```python
from build123d import *

# Parameters (mm, degrees)
SKETCH1_W           = 72
SKETCH1_H           = 36
BOSS_EXTRUDE1_DEPTH = 17
SKETCH2_W           = 124
SKETCH2_H           = 24
BOSS_EXTRUDE2_DEPTH = 12
SKETCH3_W           = 30
SKETCH3_H           = 38
BOSS_EXTRUDE3_DEPTH = 15
SKETCH4_W           = 56
SKETCH4_H           = 34
BOSS_EXTRUDE4_DEPTH = 17
SKETCH5_W           = 38
SKETCH5_H           = 18
CUT_EXTRUDE1_DEPTH  = 10
SKETCH6_R           = 7.25
CUT_EXTRUDE2_DEPTH  = 334.282162739
SKETCH7_R           = 7.5
CUT_EXTRUDE3_DEPTH  = 334.282162739


with BuildPart() as part:
    # Sketch1 → Boss-Extrude1 (new, symmetric)
    with BuildSketch(Plane.XY):
        with Locations((16, 200)):
            Rectangle(SKETCH1_W, SKETCH1_H)
    extrude(amount=BOSS_EXTRUDE1_DEPTH, both=True)

    # Sketch2 → Boss-Extrude2 (add, symmetric)
    with BuildSketch(Plane.XY):
        with Locations((110, 202)):
            Rectangle(SKETCH2_W, SKETCH2_H)
    extrude(amount=BOSS_EXTRUDE2_DEPTH, both=True)

    # Sketch3 → Boss-Extrude3 (add, symmetric)
    with BuildSketch(Plane.XY):
        with Locations((183, 203)):
            Rectangle(SKETCH3_W, SKETCH3_H)
    extrude(amount=BOSS_EXTRUDE3_DEPTH, both=True)

    # Sketch4 → Boss-Extrude4 (add, symmetric)
    with BuildSketch(Plane.XY):
        with Locations((220, 203)):
            Rectangle(SKETCH4_W, SKETCH4_H)
    extrude(amount=BOSS_EXTRUDE4_DEPTH, both=True)

    # Sketch5 → Cut-Extrude1 (cut, symmetric)
    with BuildSketch(Plane.XY):
        with Locations((233, 203)):
            Rectangle(SKETCH5_W, SKETCH5_H)
    extrude(amount=CUT_EXTRUDE1_DEPTH, both=True, mode=Mode.SUBTRACT)

    # Sketch6 → Cut-Extrude2 (cut, through all)
    with BuildSketch(Plane.XY):
        with Locations((0, 198)):
            Circle(SKETCH6_R)
    extrude(amount=-CUT_EXTRUDE2_DEPTH, mode=Mode.SUBTRACT)

    # Sketch7 → Cut-Extrude3 (cut, through all)
    with BuildSketch(Plane.XY):
        with Locations((110, 202)):
            Circle(SKETCH7_R)
    extrude(amount=-CUT_EXTRUDE3_DEPTH, mode=Mode.SUBTRACT)


solid = part.part
```
Verification items for the finished model (mm, model axes). A direction names the side the tool comes from. Give positions to 0.01 mm unless a question says otherwise; leave off trailing zeros. Loops run counter-clockwise (first coordinate to the right, second up) from the corner with the lowest first, then second, coordinate; pieces in that order, holes last. Notation, with made-up numbers: M -2,4 L 17,4 A24 ccw 17,40 Z; hole C 50,36 d7. An arc over 180 degrees is marked long. One line per question, with ' | ' between items.
Item 1: Section check C-C, the plane y = 202. Record the cut outline in (x, z).
Completed:
outline: M -20,-17 L -6.05,-17 L -6.05,0 L 6.05,0 L 6.05,-17 L 52,-17 L 52,-12 L 102.5,-12 L 102.5,0 L 117.5,0 L 117.5,-12 L 168,-12 L 168,-15 L 192,-15 L 192,-17 L 248,-17 L 248,-10 L 214,-10 L 214,10 L 248,10 L 248,17 L 192,17 L 192,15 L 168,15 L 168,12 L 52,12 L 52,17 L -20,17 Z
Item 2: Depth check by flat-ended pin: P1, Ø6, axis at x = 143.5, z = -4.5, coming from the -Y side; P2, Ø12, axis at x = 100, y = 202, coming from the +Z side; P3, Ø1, axis at x = 69, y = 204, coming from the -Z side. Enter the tip coordinate at first touch or a pass-through.
Completed:
P1: stops at y = 190 | P2: stops at z = 12 | P3: stops at z = -12
Item 3: Draft check along Z on faces 4 (the face through (15, 182, 0)), 5 (the face through (231, 203, 10)), 6 (the face through (220, 203, -17)). Enter one of: +Z half, -Z half, draft (parallel to the pull), parting line (faces both ways), or undercut.
Completed:
face 4: draft | face 5: undercut | face 6: -Z half
Item 4: Tool access check on faces 1 (the face through (109, 202, 12)), 2 (the face through (214, 203, 0)), 3 (the face through (52, 188, 0)). Record the directions out of +Z, -Z, +X, -X, +Y, -Y that give a thin tool (end or side, any length) a straight path to the whole face; none if there is none.
Completed:
face 1: +Z, +Y, -Y | face 2: +X | face 3: none
Item 5: Thickness scan on line 1 (Y direction, x = 110, z = -2.25); line 2 (X direction, y = 199.5, z = 13.5); line 3 (X direction, y = 209.5, z = -15.5). Record the ranges inside material, lowest first. Write a range as [from, to].
Completed:
line 1: y = [190, 194.5], [209.5, 214] | line 2: x = [-20, 52], [168, 248] | line 3: x = [-20, 52], [192, 248]
Item 6: Section check B-B, the plane z = 5. Record the cut outline in (x, y).
Completed:
outline: M -20,182 L 52,182 L 52,190 L 168,190 L 168,184 L 198,184 L 198,186 L 248,186 L 248,194 L 214,194 L 214,212 L 248,212 L 248,220 L 198,220 L 198,222 L 168,222 L 168,214 L 52,214 L 52,218 L -20,218 Z
Item 7: Section check A-A, the plane x = 0. Record the cut outline in (y, z).
Completed:
outline: M 182,-17 L 190.75,-17 L 190.75,0 L 205.25,0 L 205.25,-17 L 218,-17 L 218,17 L 182,17 Z
Item 8: Section check D-D, the plane x = 110. Record the cut outline in (y, z).
Completed:
outline: M 190,-12 L 194.5,-12 L 194.5,0 L 209.5,0 L 209.5,-12 L 214,-12 L 214,12 L 190,12 Z
